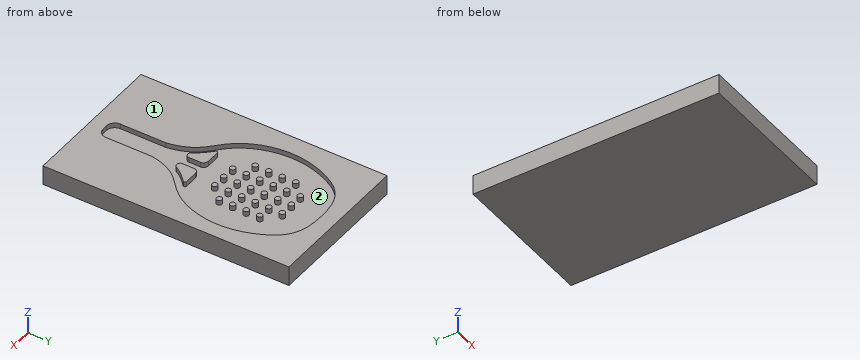
```python
from build123d import *

# Parameters (mm, degrees)
SCHIZZO1_W                   = 300
SCHIZZO1_H                   = 500
ESTRUSIONE_ESTRUSIONE1_DEPTH = 40
CAVIT_1_START                = 30
CAVIT_1_OUTLINE_R            = 5.5
CAVIT_1_DEPTH                = 10


# Read off the part's stored shape, not the designer's step: Cavità1
with BuildPart() as part:
    # Schizzo1 → Estrusione-Estrusione1 (new body)
    with BuildSketch(Plane.XY):
        with Locations((-50, 50)):
            Rectangle(SCHIZZO1_W, SCHIZZO1_H)
    extrude(amount=ESTRUSIONE_ESTRUSIONE1_DEPTH)

    # Cavità1 outline → Cavità1 (cut)
    with BuildSketch(Plane.XY.offset(CAVIT_1_START)):
        with BuildLine():
            add(Edge.make_bspline(
                [(-45.630563704, 268.931224179), (-10.242824482, 269.253777995), (26.207264329, 258.769731776), (61.298997523, 197.395847805), (78.425982638, 121.642243114), (51.329454916, 37.820129659), (-8.296880797, -5.833230992), (-20.792475043, -41.327625634), (-23.630563704, -61.068775821)],
                knots=[0, 0, 0, 0, 0.150070551, 0.226928811, 0.372737193, 0.578941384, 0.665352937, 0.775034733, 0.775034733, 0.775034733, 0.775034733], degree=3))
            add(Edge.make_bspline(
                [(-45.630563704, 268.931224179), (-81.018302926, 269.253777995), (-117.468391737, 258.769731776), (-152.560124931, 197.395847805), (-169.687110046, 121.642243114), (-142.590582324, 37.820129659), (-82.96424661, -5.833230992), (-70.468652365, -41.327625634), (-67.630563704, -61.068775821)],
                knots=[0, 0, 0, 0, 0.150070551, 0.226928811, 0.372737193, 0.578941384, 0.665352937, 0.775034733, 0.775034733, 0.775034733, 0.775034733], degree=3))
            Line((-67.630563704, -61.068775821), (-67.630563704, -154.068775821))
            ThreePointArc((-67.630563704, -154.068775821), (-62.651378984, -166.089591101), (-50.630563704, -171.068775821))
            Line((-50.630563704, -171.068775821), (-40.630563704, -171.068775821))
            ThreePointArc((-40.630563704, -171.068775821), (-28.609748424, -166.089591101), (-23.630563704, -154.068775821))
            Line((-23.630563704, -154.068775821), (-23.630563704, -61.068775821))
        make_face()
        with BuildLine():
            add(Edge.make_bspline(
                [(-94.989572549, 21.153662791), (-94.15142809, 20.375950025), (-89.988702943, 16.48850239), (-84.886613244, 11.470594112), (-79.980862553, 5.858684547), (-76.768963888, 1.916853126), (-72.951216506, -3.363954472), (-70.22044574, -7.792969084), (-68.901941305, -10.109702474)],
                knots=[0.623558075, 0.623558075, 0.623558075, 0.623558075, 0.629715721, 0.653935556, 0.659990515, 0.666045474, 0.678155392, 0.690959257, 0.690959257, 0.690959257, 0.690959257], degree=3))
            ThreePointArc((-94.989572549, 21.153662791), (-95.741625635, 24.448829767), (-92.949014353, 26.352781308))
            Line((-92.949014353, 26.352781308), (-65.630943606, 26.352781308))
            ThreePointArc((-65.630943606, 26.352781308), (-58.559875794, 23.42384912), (-55.630943606, 16.352781308))
            Line((-55.630943606, 16.352781308), (-55.630943606, -6.647312588))
            ThreePointArc((-55.630943606, -6.647312588), (-57.681196138, -11.597060056), (-62.630943606, -13.647312588))
            Line((-62.630943606, -13.647312588), (-62.818204273, -13.647312588))
            ThreePointArc((-62.818204273, -13.647312588), (-66.336959081, -12.69862357), (-68.901941305, -10.109702474))
        make_face(mode=Mode.SUBTRACT)
        with BuildLine():
            ThreePointArc((1.687854421, 26.352781308), (4.480467254, 24.448825814), (3.728406391, 21.153657015))
            add(Edge.make_bspline(
                [(3.728406391, 21.153657015), (2.890265485, 20.375951961), (-1.272467578, 16.488519054), (-6.374568867, 11.470628296), (-11.280339412, 5.858728651), (-14.492251846, 1.916903523), (-18.310034758, -3.363921174), (-21.040833914, -7.792957432), (-22.359358711, -10.109715267)],
                knots=[0.623558123, 0.623558123, 0.623558123, 0.623558123, 0.629715721, 0.653935556, 0.659990515, 0.666045474, 0.678155392, 0.690959399, 0.690959399, 0.690959399, 0.690959399], degree=3))
            ThreePointArc((-22.359358711, -10.109715267), (-24.924340017, -12.69862727), (-28.443088463, -13.647312588))
            Line((-28.443088463, -13.647312588), (-28.630183802, -13.647312588))
            ThreePointArc((-28.630183802, -13.647312588), (-33.57993127, -11.597060056), (-35.630183802, -6.647312588))
            Line((-35.630183802, -6.647312588), (-35.630183802, 16.352781308))
            ThreePointArc((-35.630183802, 16.352781308), (-32.701251613, 23.423849119), (-25.630183802, 26.352781308))
            Line((-25.630183802, 26.352781308), (1.687854421, 26.352781308))
        make_face(mode=Mode.SUBTRACT)
        with Locations((-100.630563704, 98.138648944)):
            Circle(CAVIT_1_OUTLINE_R, mode=Mode.SUBTRACT)
        with Locations((-73.130563704, 70.638648944)):
            Circle(CAVIT_1_OUTLINE_R, mode=Mode.SUBTRACT)
        with Locations((-45.630563704, 70.638648944)):
            Circle(CAVIT_1_OUTLINE_R, mode=Mode.SUBTRACT)
        with Locations((-73.130563704, 98.138648944)):
            Circle(CAVIT_1_OUTLINE_R, mode=Mode.SUBTRACT)
        with Locations((-45.630563704, 98.138648944)):
            Circle(CAVIT_1_OUTLINE_R, mode=Mode.SUBTRACT)
        with Locations((-100.630563704, 125.638648944)):
            Circle(CAVIT_1_OUTLINE_R, mode=Mode.SUBTRACT)
        with Locations((-100.630563704, 153.138648944)):
            Circle(CAVIT_1_OUTLINE_R, mode=Mode.SUBTRACT)
        with Locations((-73.130563704, 125.638648944)):
            Circle(CAVIT_1_OUTLINE_R, mode=Mode.SUBTRACT)
        with Locations((-45.630563704, 125.638648944)):
            Circle(CAVIT_1_OUTLINE_R, mode=Mode.SUBTRACT)
        with Locations((-73.130563704, 153.138648944)):
            Circle(CAVIT_1_OUTLINE_R, mode=Mode.SUBTRACT)
        with Locations((-45.630563704, 153.138648944)):
            Circle(CAVIT_1_OUTLINE_R, mode=Mode.SUBTRACT)
        with Locations((-100.630563704, 180.638648944)):
            Circle(CAVIT_1_OUTLINE_R, mode=Mode.SUBTRACT)
        with Locations((-73.130563704, 180.638648944)):
            Circle(CAVIT_1_OUTLINE_R, mode=Mode.SUBTRACT)
        with Locations((-45.630563704, 180.638648944)):
            Circle(CAVIT_1_OUTLINE_R, mode=Mode.SUBTRACT)
        with Locations((-73.130563704, 208.138648944)):
            Circle(CAVIT_1_OUTLINE_R, mode=Mode.SUBTRACT)
        with Locations((-45.630563704, 208.138648944)):
            Circle(CAVIT_1_OUTLINE_R, mode=Mode.SUBTRACT)
        with Locations((-18.130563704, 70.638648944)):
            Circle(CAVIT_1_OUTLINE_R, mode=Mode.SUBTRACT)
        with Locations((-18.130563704, 98.138648944)):
            Circle(CAVIT_1_OUTLINE_R, mode=Mode.SUBTRACT)
        with Locations((9.369436296, 98.138648944)):
            Circle(CAVIT_1_OUTLINE_R, mode=Mode.SUBTRACT)
        with Locations((-18.130563704, 125.638648944)):
            Circle(CAVIT_1_OUTLINE_R, mode=Mode.SUBTRACT)
        with Locations((-18.130563704, 153.138648944)):
            Circle(CAVIT_1_OUTLINE_R, mode=Mode.SUBTRACT)
        with Locations((9.369436296, 125.638648944)):
            Circle(CAVIT_1_OUTLINE_R, mode=Mode.SUBTRACT)
        with Locations((9.369436296, 153.138648944)):
            Circle(CAVIT_1_OUTLINE_R, mode=Mode.SUBTRACT)
        with Locations((-18.130563704, 180.638648944)):
            Circle(CAVIT_1_OUTLINE_R, mode=Mode.SUBTRACT)
        with Locations((-18.130563704, 208.138648944)):
            Circle(CAVIT_1_OUTLINE_R, mode=Mode.SUBTRACT)
        with Locations((9.369436296, 180.638648944)):
            Circle(CAVIT_1_OUTLINE_R, mode=Mode.SUBTRACT)
    extrude(amount=CAVIT_1_DEPTH, mode=Mode.SUBTRACT)


solid = part.part
```
CAD build for the part. Positions are in the model's coordinates, mm. Face numbers are marked on the shaded views. Round coordinates to 2 decimals unless told otherwise and drop trailing zeros. Loops run counter-clockwise (first coordinate to the right, second up) from the corner with the lowest first, then second, coordinate; pieces in that order, holes last. Notation, with made-up numbers: M 70,-19 L 103,-19 A15 cw 103,-14 Z; hole C -35,25 d6. An arc over 180 degrees is marked long. Return JSON: item names as keys, results as strings. Group by question number.
(1) Wall check: probe 1 along Y at (x, z) = (-10, 35.5); probe 2 along Z at (x, y) = (9, 59.5); probe 3 along X at (y, z) = (187.5, 34.5). Give the ranges that are in metal, low to high. Write a range as [from, to].
(2) Saw through at A-A, the plane y = -75.5. List the corners of the cut face in (x, z), and give its area (3 significant figures).
(3) Mould opens along Y. For the marked faces 1 and 2 say: +Y half, -Y half, draft (parallel to the pull), parting line (faces both ways), or undercut.
Answer list:
{
 "1": {"probe 1": "[-200, -18.74], [7.32, 26.35], [265.93, 300]", "probe 2": "[0, 30]", "probe 3": "[-200, -152.63], [61.37, 100]"},
 "2": {"outline": "M -200,0 L 100,0 L 100,40 L -23.63,40 L -23.63,30 L -67.63,30 L -67.63,40 L -200,40 Z", "area": "11,600 mm2"},
 "3": {"face 1": "draft", "face 2": "undercut"}
}
